Check sheet for the drawn part. Datum: minimum x, y, z corner. Units: mm. Round coordinates to 2 decimals unless told otherwise and drop trailing zeros. Write each loop counter-clockwise with the first axis right and the second up, starting at its lowest first coordinate (ties: lowest second). Pieces come first, ordered by that corner, then holes.
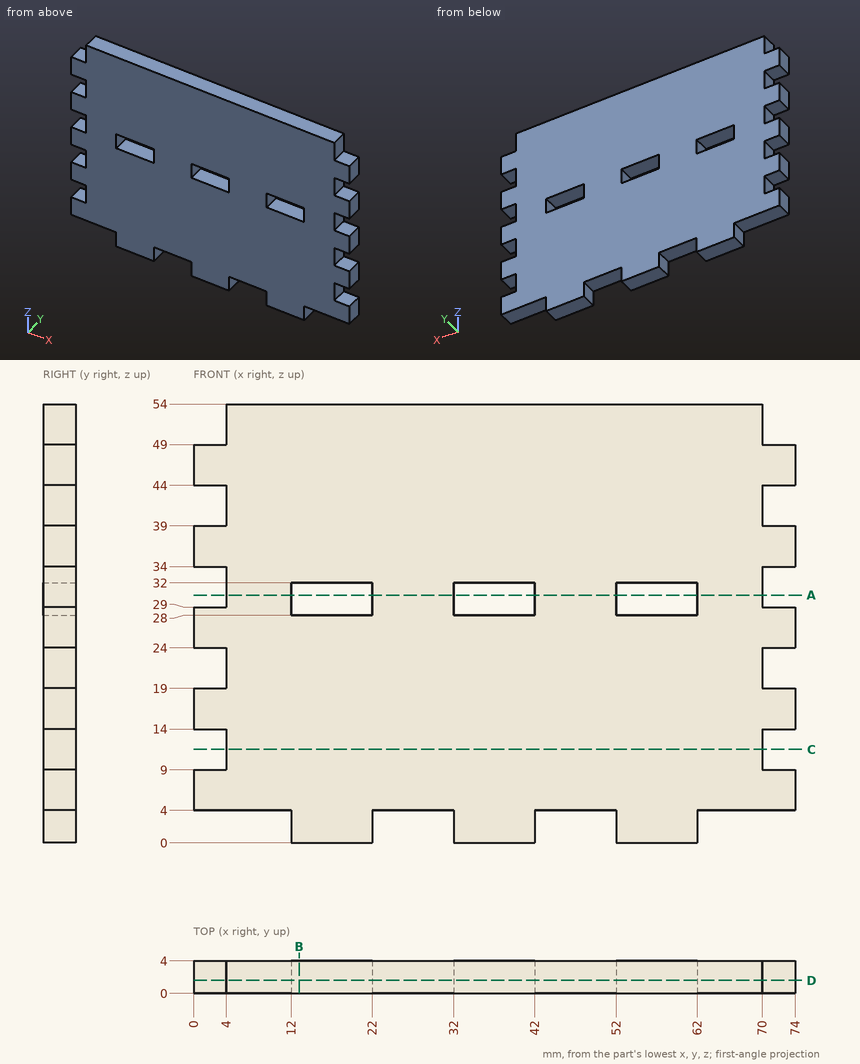
Q1. Sectioned sample at B-B (x = 13). Enter the section's corners in (y, z).
Recorded:
outline: (0, 0) - (4, 0) - (4, 28) - (0, 28) - close; (0, 32) - (4, 32) - (4, 54) - (0, 54) - close
Q2. Sectioned sample at C-C (z = 11.5). Enter the section's corners in (x, y).
Recorded:
outline: (4, 0) - (70, 0) - (70, 4) - (4, 4) - close
Q3. Depth check by flat-ended pin: P1, Ø1.2, axis at y = 1.5, z = 31, coming from the -X side; P2, Ø1.2, axis at y = 1.5, z = 1.5, coming from the -X side; P3, Ø1.2, axis at x = 2, y = 2, coming from the +Z side; P4, Ø2, axis at x = 58, z = 34, coming from the -Y side. Enter the tip coordinate at first touch or a pass-through.
Recorded:
P1: stops at x = 4
P2: stops at x = 12
P3: stops at z = 49
P4: stops at y = 0
Q4. Sectioned sample at A-A (z = 30.5). Enter the section's corners in (x, y).
Recorded:
outline: (4, 0) - (12, 0) - (12, 4) - (4, 4) - close; (22, 0) - (32, 0) - (32, 4) - (22, 4) - close; (42, 0) - (52, 0) - (52, 4) - (42, 4) - close; (62, 0) - (70, 0) - (70, 4) - (62, 4) - close
Q5. Sectioned sample at D-D (y = 1.6). Give the number of separate pieces and of enclosed holes in the cut face, plus the area to 3 significant figures.
Recorded:
separate pieces: 1
enclosed holes: 3
area: 3,500 mm2
Q6. Material ranges on line 1 along X through (y, z) = (3.35, 30); line 2 along Z through (x, y) = (61.5, 3.75); line 3 along Z through (x, y) = (29, 1.85), recorded low to high.
Recorded:
line 1: x = 4 to 12, 22 to 32, 42 to 52, 62 to 70
line 2: z = 0 to 28, 32 to 54
line 3: z = 4 to 54
